from build123d import *

# Parameters (mm, degrees)
SKETCH1_W            = 1818.96
SKETCH1_H            = 606.96
BOSS_EXTRUDE2_DEPTH  = 53.48
BOSS_EXTRUDE9_DEPTH  = 3.48
BOSS_EXTRUDE10_DEPTH = 6.96
BOSS_EXTRUDE11_START = 6.96
BOSS_EXTRUDE11_DEPTH = 3.48


with BuildPart() as part:
    # Sketch1 → Boss-Extrude2 (new body)
    with BuildSketch(Plane(origin=(0, 0, 0), x_dir=(1, 0, 0), z_dir=(0, 1, 0))):
        with Locations((906, -300)):
            Rectangle(SKETCH1_W, SKETCH1_H)
        Polygon((274.507750304, 0), (0, -600), (0, 0), align=None, mode=Mode.SUBTRACT)
        Polygon((3.826921158, -600), (278.334671461, 0), (325.665328539, 0), (600.173078842, -600), align=None, mode=Mode.SUBTRACT)
        Polygon((607.826921158, -600), (882.334671461, 0), (929.665328539, 0), (1204.173078842, -600), align=None, mode=Mode.SUBTRACT)
        Polygon((1211.826921158, -600), (1486.334671461, 0), (1533.665328539, 0), (1808.173078842, -600), align=None, mode=Mode.SUBTRACT)
        Polygon((1812, 0), (1812, -600), (1537.492249696, 0), align=None, mode=Mode.SUBTRACT)
        Polygon((933.492249696, 0), (1482.507750304, 0), (1208, -600), align=None, mode=Mode.SUBTRACT)
        Polygon((329.492249696, 0), (878.507750304, 0), (604, -600), align=None, mode=Mode.SUBTRACT)
    extrude(amount=BOSS_EXTRUDE2_DEPTH)

    # Sketch1<7> → Boss-Extrude9 (add)
    with BuildSketch(Plane(origin=(0, 0, 0), x_dir=(1, 0, 0), z_dir=(0, 1, 0))):
        Polygon((37.337927674, -578.48), (27.492249696, -600), (576.507750304, -600), (566.662072326, -578.48), align=None)
        Polygon((274.507750304, 0), (0, 0), (0, -600), (21.52, -552.963076686), (21.52, -21.52), (264.662072326, -21.52), align=None)
        Polygon((641.337927674, -578.48), (631.492249696, -600), (1180.507750304, -600), (1170.662072326, -578.48), align=None)
        Polygon((1245.337927674, -578.48), (1235.492249696, -600), (1784.507750304, -600), (1774.662072326, -578.48), align=None)
        Polygon((1812, 0), (1537.492249696, 0), (1547.337927674, -21.52), (1790.48, -21.52), (1790.48, -552.963076686), (1812, -600), align=None)
        Polygon((1198.154322022, -578.48), (1208, -600), (1217.845677978, -578.48), align=None)
        Polygon((594.154322022, -578.48), (604, -600), (613.845677978, -578.48), align=None)
        Polygon((1482.507750304, 0), (933.492249696, 0), (943.337927674, -21.52), (1472.662072326, -21.52), align=None)
        Polygon((1519.845677978, -21.52), (1510, 0), (1500.154322022, -21.52), align=None)
        Polygon((915.845677978, -21.52), (906, 0), (896.154322022, -21.52), align=None)
        Polygon((878.507750304, 0), (329.492249696, 0), (339.337927674, -21.52), (868.662072326, -21.52), align=None)
        Polygon((311.845677978, -21.52), (302, 0), (292.154322022, -21.52), align=None)
    extrude(amount=BOSS_EXTRUDE9_DEPTH)

    # Sketch1<9> → Boss-Extrude10 (add)
    with BuildSketch(Plane(origin=(0, 0, 0), x_dir=(1, 0, 0), z_dir=(0, 1, 0))):
        Polygon((1774.662072326, -578.48), (1784.507750304, -600), (1808.173078842, -600), (1790.48, -561.327695507), (1790.48, -578.48), align=None)
        Polygon((1221.672599135, -578.48), (1211.826921158, -600), (1235.492249696, -600), (1245.337927674, -578.48), align=None)
        Polygon((1170.662072326, -578.48), (1180.507750304, -600), (1204.173078842, -600), (1194.327400865, -578.48), align=None)
        Polygon((617.672599135, -578.48), (607.826921158, -600), (631.492249696, -600), (641.337927674, -578.48), align=None)
        Polygon((566.662072326, -578.48), (576.507750304, -600), (600.173078842, -600), (590.327400865, -578.48), align=None)
        Polygon((21.52, -561.327695507), (3.826921158, -600), (27.492249696, -600), (37.337927674, -578.48), (21.52, -578.48), align=None)
        Polygon((302, 0), (278.334671461, 0), (268.488993484, -21.52), (292.154322022, -21.52), align=None)
        Polygon((325.665328539, 0), (302, 0), (311.845677978, -21.52), (335.511006516, -21.52), align=None)
        Polygon((929.665328539, 0), (906, 0), (915.845677978, -21.52), (939.511006516, -21.52), align=None)
        Polygon((906, 0), (882.334671461, 0), (872.488993484, -21.52), (896.154322022, -21.52), align=None)
        Polygon((1533.665328539, 0), (1510, 0), (1519.845677978, -21.52), (1543.511006516, -21.52), align=None)
        Polygon((1510, 0), (1486.334671461, 0), (1476.488993484, -21.52), (1500.154322022, -21.52), align=None)
    extrude(amount=BOSS_EXTRUDE10_DEPTH)

    # Sketch1<10> → Boss-Extrude11 (add)
    with BuildSketch(Plane(origin=(0, 0, 0), x_dir=(1, 0, 0), z_dir=(0, 1, 0)).offset(BOSS_EXTRUDE11_START)):
        Polygon((292.154322022, -21.52), (268.488993484, -21.52), (21.52, -561.327695507), (21.52, -578.48), (37.337927674, -578.48), align=None)
        Polygon((335.511006516, -21.52), (311.845677978, -21.52), (566.662072326, -578.48), (590.327400865, -578.48), align=None)
        Polygon((896.154322022, -21.52), (872.488993484, -21.52), (617.672599135, -578.48), (641.337927674, -578.48), align=None)
        Polygon((939.511006516, -21.52), (915.845677978, -21.52), (1170.662072326, -578.48), (1194.327400865, -578.48), align=None)
        Polygon((1500.154322022, -21.52), (1476.488993484, -21.52), (1221.672599135, -578.48), (1245.337927674, -578.48), align=None)
        Polygon((1543.511006516, -21.52), (1519.845677978, -21.52), (1774.662072326, -578.48), (1790.48, -578.48), (1790.48, -561.327695507), align=None)
    extrude(amount=-BOSS_EXTRUDE11_DEPTH)


solid = part.part
The listing builds one solid part. Answer for the finished solid, in the listing's coordinates (mm). A direction names the side the tool comes from. Round coordinates to 2 decimals unless told otherwise and drop trailing zeros. Write each loop counter-clockwise with the first axis right and the second up, starting at its lowest first coordinate (ties: lowest second). Pieces come first, ordered by that corner, then holes. Notation, with made-up numbers: M 70.25,77.5 L 124.25,77.5 A23 cw 124.25,111.5 Z; hole C 23.25,53.5 d10. An arc over 180 degrees is marked long. Write each question's results on one line, items separated by ' | '. Start each with the question number.
Item 1: Which of the six approach directions +Z, -Z, +X, -X, +Y, -Y give full straight-line access (tool end or side, diameter ignored) to faces 4 (the flat face through (1673, 28, 0)), 5 (the flat face through (450, 3.48, 299))?
Item 2: Given pin 1 Ø21.5 at (x, z) = (1211, 589.5) entering from +Y; pin 2 Ø17 at (x, z) = (1200.5, 14) entering from +Y; pin 3 Ø16 at (x, z) = (901.5, 11) entering from +Y, each flat-ended and moving along its own axis, determine where each tip first touches the part or whether it passes through.
Item 3: Find section B-B on x = 1423. Write down the section's boundary in (y, z), and give its area (3 significant figures).
Item 4: Straight lines are drawn through the part: probe 1 along Z at (x, y) = (627, 45.5); probe 2 along Z at (x, y) = (929, 16); probe 3 along Z at (x, y) = (1320.5, 36). For each, find the intervals that lie inside material, in ascending order.
Item 5: The mould has two halves that part along X. Classify faces 1 (the flat face through (1812, 28, 296)), 2 (the flat face through (-3.48, 26, 304)), 3 (the flat face through (1815.48, 26, 304)): +X half, -X half, draft (parallel to the pull), parting line (faces both ways), or undercut.
Item 6: Find section A-A on y = 33.5. Write down the section's boundary in (x, z), and give its area (3 significant figures).
Item 7: Find section C-C on z = 484.5. Give the number of separate pieces and of enclosed holes in the cut face, and give its area (3 significant figures).
Answer block:
1) face 4: +Y | face 5: -Y
2) pin 1: stops at y = 53.48 | pin 2: stops at y = 3.48 | pin 3: stops at y = 6.96
3) outline: M 0,-3.48 L 53.48,-3.48 L 53.48,0 L 3.48,0 L 3.48,21.52 L 0,21.52 Z; M 0,130.07 L 53.48,130.07 L 53.48,138.43 L 6.96,138.43 L 6.96,190.16 L 3.48,190.16 L 3.48,138.43 L 0,138.43 Z; M 0,578.48 L 3.48,578.48 L 3.48,600 L 53.48,600 L 53.48,603.48 L 0,603.48 Z | area: 1,150 mm²
4) probe 1: z = -3.48 to 0, 549.73 to 558.09, 600 to 603.48 | probe 2: z = -3.48 to 0, 600 to 603.48 | probe 3: z = -3.48 to 0, 354.11 to 362.47, 600 to 603.48
5) face 1: undercut | face 2: -X half | face 3: +X half
6) outline: M -3.48,-3.48 L 1815.48,-3.48 L 1815.48,603.48 L -3.48,603.48 Z; hole M 0,0 L 274.51,0 L 0,600 Z; hole M 3.83,600 L 278.33,0 L 325.67,0 L 600.17,600 Z; hole M 329.49,0 L 878.51,0 L 604,600 Z; hole M 607.83,600 L 882.33,0 L 929.67,0 L 1204.17,600 Z; hole M 933.49,0 L 1482.51,0 L 1208,600 Z; hole M 1211.83,600 L 1486.33,0 L 1533.67,0 L 1808.17,600 Z; hole M 1537.49,0 L 1812,0 L 1812,600 Z | area: 30,600 mm²
7) separate pieces: 8 | enclosed holes: 0 | area: 2,240 mm²
